Geometry check sheet. Reference: the model listing, model coordinates, mm. Face numbers are marked on the shaded views. A direction names the side the tool comes from. Round coordinates to 2 decimals unless told otherwise and drop trailing zeros. Order: outer loops, then holes, each group sorted by start corner. A loop starts at its lowest first (then second) coordinate and runs counter-clockwise, first axis right, second up. Notation, with made-up numbers: (70, -33.5) -> (107, -33.5) arc R21 ccw to (107, -22.5) -> close; hole circle Ø9 at (47, 82.5). An arc over 180 degrees is marked (long way). Use a Markdown table: item, result. Add a question column.
Item 1: Sectioned sample at D-D, the plane z = 63.5. Record the cut outline in (x, y), and give its area (3 significant figures).
Item 2: Set-up check for the marked faces 1, 2 and 3: record each of +Z, -Z, +X, -X, +Y, -Y from which the full face is reachable in a straight line by a thin tool's end or side.
Item 3: Sectioned sample at B-B, the plane z = 30. State how many separate pieces and enclosed holes the cut face has, and give its area (3 significant figures).
Item 4: Gauge pin test, flat ends, axial feed: pin 1 Ø1.5 at (x, y) = (10.5, -93.5) entering from +Z; pin 2 Ø10.5 at (x, z) = (13.5, 33.5) entering from +Y; pin 3 Ø3 at (x, z) = (13.5, 63.5) entering from +Y; pin 4 Ø1.5 at (y, z) = (-70.5, 40.5) entering from -X. Record the tip position at first contact, or that the pin passes through.
Item 5: Sectioned sample at A-A, the plane y = -15. Record the cut outline in (x, z) (3 decimals).
Item 6: Sectioned sample at C-C, the plane x = 30. Record the cut outline in (y, z), and give its area (3 significant figures).
Item 7: Material ranges on probe 1 along X at (y, z) = (-2, 31); probe 2 along Z at (x, y) = (24.5, -101.5); probe 3 along X at (y, z) = (-22, 5) (3 decimals), recorded low to high. Write a range as [from, to].
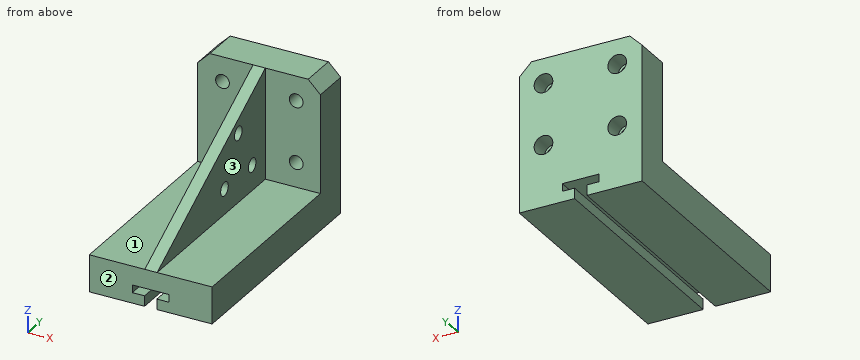
from build123d import *

# Parameters (mm, degrees)
F1_DEPTH       = 19.05
F3_W           = 63.5
F3_H           = 19.05
F4_DEPTH       = 120.65
F5_DEPTH       = 120.65
F7_D           = 7.112
F7_CBORE_D     = 9.652
F7_CBORE_DEPTH = 9.652
F9_START       = 28.702
F9_DEPTH       = 6.35
F11_D          = 7.112
F11_DEPTH      = 12.7
F11_TIP        = 2.1366603613


with BuildPart() as f1:
    # F0 (on Front) → F1 (new body)
    with BuildSketch(Plane.XZ):
        Polygon((6.35, 76.2), (0, 69.85), (0, 0), (63.5, 0), (63.5, 69.85), (57.15, 76.2), align=None)
    extrude(amount=F1_DEPTH)

    # F3 (on Front) → F4 (join)
    with BuildSketch(Plane.XZ):
        with Locations((31.75, 9.525)):
            Rectangle(F3_W, F3_H)
    extrude(amount=F4_DEPTH)

    # F2 (on Front) → F5 (cut)
    with BuildSketch(Plane.XZ):
        Polygon((28.575, 0), (34.925, 0), (34.925, 5.3848), (41.275, 5.3848), (41.275, 9.3472), (22.225, 9.3472), (22.225, 5.3848), (28.575, 5.3848), align=None)
    extrude(amount=F5_DEPTH, mode=Mode.SUBTRACT)

    # F7 (through all)
    with Locations(Plane(origin=(0, 0, 0), x_dir=(-1, 0, 0), z_dir=(0, 1, 0))):
        with Locations((-50.9831043839, 63.5), (-12.8831043839, 63.5), (-12.8831043839, 31.75), (-50.9831043839, 31.75)):
            CounterBoreHole(F7_D / 2, F7_CBORE_D / 2, F7_CBORE_DEPTH)

    # F8 (on Right) → F9 (join)
    with BuildSketch(Plane.YZ.offset(F9_START)):
        Polygon((-19.05, 76.2), (-120.65, 19.05), (-19.05, 19.05), align=None)
    extrude(amount=F9_DEPTH)

    # F11
    with Locations(Plane.YZ.offset(35.052)):
        with Locations((-44.45, 54.61), (-31.4717432989, 32.131), (-57.4282567011, 32.131)):
            Hole(F11_D / 2, depth=F11_DEPTH)
            with Locations((0, 0, -(F11_DEPTH + F11_TIP / 2))):  # 118° drill point
                Cone(0, F11_D / 2, F11_TIP, mode=Mode.SUBTRACT)


solid = f1.part
Found:
| question | item | result |
|---|---|---|
| 1 | outline | (0, -19.05) -> (9.33, -19.05) -> (9.33, -9.65) -> (8.06, -9.65) -> (8.06, 0) -> (0, 0) -> close; (16.44, -19.05) -> (28.7, -19.05) -> (28.7, -41.63) -> (35.05, -41.63) -> (35.05, -19.05) -> (47.43, -19.05) -> (47.43, -9.65) -> (46.16, -9.65) -> (46.16, 0) -> (17.71, 0) -> (17.71, -9.65) -> (16.44, -9.65) -> close; (54.54, -19.05) -> (63.5, -19.05) -> (63.5, 0) -> (55.81, 0) -> (55.81, -9.65) -> (54.54, -9.65) -> close |
| 1 | area | 1,030 mm2 |
| 2 | face 1 | +Z, -X, -Y |
| 2 | face 2 | +Z, -Z, +X, -X, -Y |
| 2 | face 3 | +Z, +X, -Y |
| 3 | separate pieces | 5 |
| 3 | enclosed holes | 0 |
| 3 | area | 1,370 mm2 |
| 4 | pin 1 | stops at z = 19.05 |
| 4 | pin 2 | stops at y = 0 |
| 4 | pin 3 | passes through |
| 4 | pin 4 | stops at x = 28.7 |
| 5 | outline | (0, 0) -> (28.575, 0) -> (28.575, 5.385) -> (22.225, 5.385) -> (22.225, 9.347) -> (41.275, 9.347) -> (41.275, 5.385) -> (34.925, 5.385) -> (34.925, 0) -> (63.5, 0) -> (63.5, 69.85) -> (57.15, 76.2) -> (6.35, 76.2) -> (0, 69.85) -> close; hole circle Ø7.112 at (12.883, 31.75); hole circle Ø7.112 at (12.883, 63.5); hole circle Ø7.112 at (50.983, 31.75); hole circle Ø7.112 at (50.983, 63.5) |
| 6 | outline | (-120.65, 9.35) -> (0, 9.35) -> (0, 76.2) -> (-19.05, 76.2) -> (-120.65, 19.05) -> close; hole circle Ø7.11 at (-57.43, 32.13); hole circle Ø7.11 at (-44.45, 54.61); hole circle Ø7.11 at (-31.47, 32.13) |
| 6 | area | 5,040 mm2 |
| 7 | probe 1 | x = [0, 8.12], [17.65, 46.22], [55.75, 63.5] |
| 7 | probe 2 | z = [0, 5.38], [9.35, 19.05] |
| 7 | probe 3 | x = [0, 28.575], [34.925, 63.5] |
